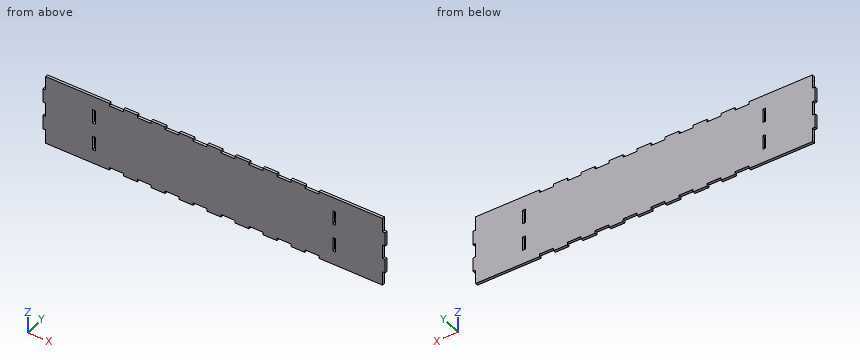
```python
from build123d import *

# Parameters (mm, degrees)
BOSS_EXTRUDE1_DEPTH = 4.826
SKETCH2_W           = 4.826
SKETCH2_H           = 25.4
CUT_EXTRUDE1_DEPTH  = 5.826
SKETCH3_W           = 25.4
SKETCH3_H           = 4.826
CUT_EXTRUDE2_DEPTH  = 5.826


with BuildPart() as part:
    # Sketch1 → Boss-Extrude1 (new body)
    with BuildSketch(Plane(origin=(0, 0, 0), x_dir=(1, 0, 0), z_dir=(0, 1, 0))):
        Polygon((0, 101.6), (0, 127), (612.648, 127), (612.648, 101.6), (617.474, 101.6), (617.474, 76.2), (612.648, 76.2), (612.648, 50.8), (617.474, 50.8), (617.474, 25.4), (612.648, 25.4), (612.648, 0), (0, 0), (0, 25.4), (-4.826, 25.4), (-4.826, 50.8), (0, 50.8), (0, 76.2), (-4.826, 76.2), (-4.826, 101.6), align=None)
    extrude(amount=BOSS_EXTRUDE1_DEPTH)

    # Sketch2 → Cut-Extrude1 (cut, through all)
    with BuildSketch(Plane(origin=(0, 4.826, 0), x_dir=(1, 0, 0), z_dir=(0, 1, 0))):
        with Locations((524.637, 88.9)):
            Rectangle(SKETCH2_W, SKETCH2_H)
        with Locations((524.637, 38.1)):
            Rectangle(SKETCH2_W, SKETCH2_H)
        with Locations((88.011, 38.1)):
            Rectangle(SKETCH2_W, SKETCH2_H)
        with Locations((88.011, 88.9)):
            Rectangle(SKETCH2_W, SKETCH2_H)
    extrude(amount=-CUT_EXTRUDE1_DEPTH, mode=Mode.SUBTRACT)

    # Sketch3 → Cut-Extrude2 (cut, through all)
    with BuildSketch(Plane(origin=(0, 4.826, 0), x_dir=(1, 0, 0), z_dir=(0, 1, 0))):
        with Locations((484.124, 2.413)):
            Rectangle(SKETCH3_W, SKETCH3_H)
        with Locations((433.324, 2.413)):
            Rectangle(SKETCH3_W, SKETCH3_H)
        with Locations((382.524, 2.413)):
            Rectangle(SKETCH3_W, SKETCH3_H)
        with Locations((331.724, 2.413)):
            Rectangle(SKETCH3_W, SKETCH3_H)
        with Locations((280.924, 2.413)):
            Rectangle(SKETCH3_W, SKETCH3_H)
        with Locations((230.124, 2.413)):
            Rectangle(SKETCH3_W, SKETCH3_H)
        with Locations((128.524, 2.413)):
            Rectangle(SKETCH3_W, SKETCH3_H)
        with Locations((179.324, 2.413)):
            Rectangle(SKETCH3_W, SKETCH3_H)
        with Locations((128.524, 124.587)):
            Rectangle(SKETCH3_W, SKETCH3_H)
        with Locations((179.324, 124.587)):
            Rectangle(SKETCH3_W, SKETCH3_H)
        with Locations((230.124, 124.587)):
            Rectangle(SKETCH3_W, SKETCH3_H)
        with Locations((280.924, 124.587)):
            Rectangle(SKETCH3_W, SKETCH3_H)
        with Locations((331.724, 124.587)):
            Rectangle(SKETCH3_W, SKETCH3_H)
        with Locations((382.524, 124.587)):
            Rectangle(SKETCH3_W, SKETCH3_H)
        with Locations((433.324, 124.587)):
            Rectangle(SKETCH3_W, SKETCH3_H)
        with Locations((484.124, 124.587)):
            Rectangle(SKETCH3_W, SKETCH3_H)
    extrude(amount=-CUT_EXTRUDE2_DEPTH, mode=Mode.SUBTRACT)


solid = part.part
```
The model under review builds one solid part; all positions refer to its coordinate system, in mm. Coordinates: 2 decimals unless noted, no trailing zeros. Write each loop counter-clockwise with the first axis right and the second up, starting at its lowest first coordinate (ties: lowest second). Pieces come first, ordered by that corner, then holes.
1) We need section A-A on z = -34.5. State the section outline as (x, y) points.
2) To check wall thickness, follow probe 1 along X at (y, z) = (4, -99); probe 2 along X at (y, z) = (0.2, -105); probe 3 along Z at (x, y) = (232, 3.7). State the ranges of each line that lie inside material, in increasing order.
3) Clearance check with flat-ended pins moving along their axes: pin 1 Ø1.4 at (y, z) = (3, -125.5) entering from +X; pin 2 Ø1.4 at (y, z) = (2.5, -2) entering from -X; pin 3 Ø1.4 at (x, y) = (132.5, 1.5) entering from +Z. State where each tip first meets the part, or that it passes through.
4) We need section D-D on z = -117. State the section outline as (x, y) points, then the cut area to 3 significant figures.
5) We need section B-B on y = 3. Count the separate pieces of the cut face and the enclosed holes in it, then the cut area to 3 significant figures.
6) We need section C-C on x = 332. State the section outline as (y, z) points, then the cut area to 3 significant figures.
Answer list:
1. outline: (-4.83, 0) - (85.6, 0) - (85.6, 4.83) - (-4.83, 4.83) - close; (90.42, 0) - (522.22, 0) - (522.22, 4.83) - (90.42, 4.83) - close; (527.05, 0) - (617.47, 0) - (617.47, 4.83) - (527.05, 4.83) - close
2. probe 1: x = -4.83 to 85.6, 90.42 to 522.22, 527.05 to 617.47
2. probe 2: x = 0 to 612.65
2. probe 3: z = -122.17 to -4.83
3. pin 1: stops at x = 612.65
3. pin 2: stops at x = 0
3. pin 3: stops at z = -4.83
4. outline: (0, 0) - (612.65, 0) - (612.65, 4.83) - (0, 4.83) - close
4. area: 2,960 mm2
5. separate pieces: 1
5. enclosed holes: 4
5. area: 75,800 mm2
6. outline: (0, -122.17) - (4.83, -122.17) - (4.83, -4.83) - (0, -4.83) - close
6. area: 566 mm2
